Autodesk Inventor part; units mm, degrees
ref_plane "YZ Plane" through (0, 0, 0) normal (1, 0, 0) x (0, 1, 0)
ref_plane "XZ Plane" through (0, 0, 0) normal (0, 1, 0) x (-1, 0, 0)
ref_plane "XY Plane" through (0, 0, 0) normal (0, 0, 1) x (1, 0, 0)
sketch "Sketch1" plane through (0, 0, 0) normal (0, 0, 1) x (1, 0, 0)
  circle A0 centre (0, 0) radius 12.5
  circle A1 centre (0, 0) radius 21
  dimension "d0" = 25
  dimension "d1" = 42
extrude "Extrusion1" add sketch "Sketch1" along normal blind 15
fillet "Fillet1" radius 2 2 edges at (-21, 0, 15) (-21, 0, 0)
fillet "Fillet2" radius 1 2 edges at (-12.5, 0, 0) (-12.5, 0, 15)
properties part number "U51105" material "Steel, Carbon"
Geometry: final body of the model. Coordinates: model frame, mm. Give positions to 0.01 mm unless a question says otherwise; leave off trailing zeros. Order: outer loops, then holes, each group sorted by start corner. A loop starts at its lowest first (then second) coordinate and runs counter-clockwise, first axis right, second up. Notation, with made-up numbers: (62, 15.25) - (114, 15.25) arc R23 cw to (114, 38.25) - close; hole circle Ø8 at (-37.5, 42.25). An arc over 180 degrees is marked (long way). Use CSV: the item, a comma, the result in double quotes.
1. Section query A-A (y = 0). Output: boundary loops of the cut face in (x, z), plus the area to 3 significant figures.
Answers below:
outline,"(-21, 2) arc R2 ccw to (-19, 0) - (-13.5, 0) arc R1 ccw to (-12.5, 1) - (-12.5, 14) arc R1 ccw to (-13.5, 15) - (-19, 15) arc R2 ccw to (-21, 13) - close; (12.5, 1) arc R1 ccw to (13.5, 0) - (19, 0) arc R2 ccw to (21, 2) - (21, 13) arc R2 ccw to (19, 15) - (13.5, 15) arc R1 ccw to (12.5, 14) - close"
area,"251 mm2"
2. Section query C-C (z = 12). Output: boundary loops of the cut face in (x, y), plus the area to 3 significant figures.
Answers below:
outline,"circle Ø42 at (0, 0); hole circle Ø25 at (0, 0)"
area,"895 mm2"
3. Mould query, pull axis X, two halves, no side actions, for faces 1 (the face through (20.03, -6.31, 7.42)), 2 (the face through (-4.5, 12.9, 15)), 3 (the face through (11.923, -3.755, 7.409)). Classes: +X half, -X half, draft (parallel to the pull), parting line (faces both ways), or undercut.
Answers below:
face 1,"parting line"
face 2,"draft"
face 3,"undercut"
4. Contact query for flat-ended pins moving along their axis: pin 1 (3 mm diameter, centred on x = -9.5, z = 1.5, fed in from +Y); pin 2 (2 mm diameter, centred on x = 16.5, z = 9.5, fed in from +Y); pin 3 (10 mm diameter, centred on x = 7, y = 3.5, fed in from +Z). Output: stop coordinate, or through.
Answers below:
pin 1,"y = 19.39"
pin 2,"y = 14.17"
pin 3,"z = 14.74"
5. Material intervals for line 1 along Y through (x, z) = (0, 5); line 2 along Y through (x, z) = (-7, 13.75); line 3 along X through (y, z) = (4, 13.5), sorted ascending. Write a range as from..to.
Answers below:
line 1,"-21..-12.5, 12.5..21"
line 2,"-19.64..-10.36, 10.36..19.64"
line 3,"-20.55..-11.84, 11.84..20.55"
